Input: dimensioned drawing with shaded views. Units: mm. Origin: part minimum x, y, z. A direction names the side the tool comes from. Round coordinates to 2 decimals unless told otherwise and drop trailing zeros. Loops run counter-clockwise (first coordinate to the right, second up) from the corner with the lowest first, then second, coordinate; pieces in that order, holes last. Notation, with made-up numbers: (45.25, 18) - (54.25, 18) arc R28 cw to (54.25, 46) - close; hole circle Ø4 at (86.5, 70). An arc over 180 degrees is marked (long way). Answer as CSV lines item,"result".
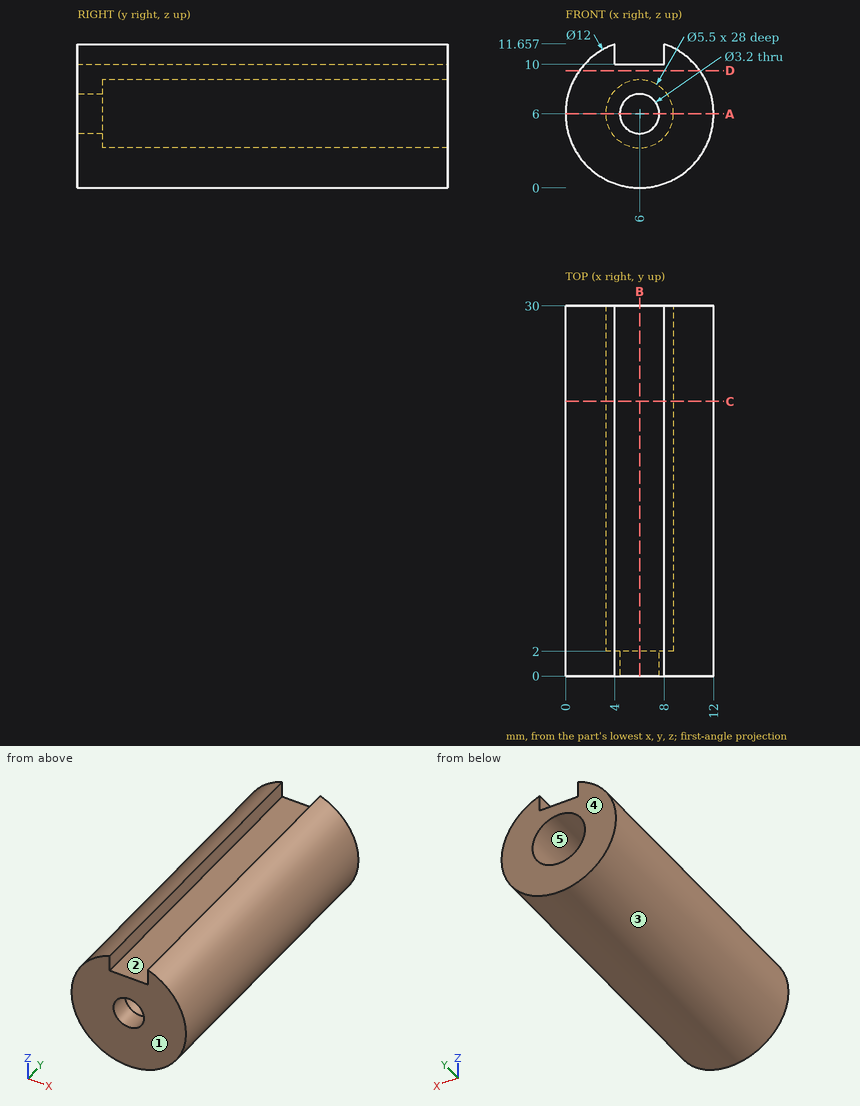
(1) Material intervals for line 1 along Z through (x, y) = (6, 1.1); line 2 along Z through (x, y) = (6, 11.5); line 3 along Y through (x, z) = (4, 7.75), sorted ascending.
Findings below:
line 1,"0 to 4.4, 7.6 to 10"
line 2,"0 to 3.25, 8.75 to 10"
line 3,"0 to 2"
(2) Pin query (flat end, axial travel): P1, Ø5, axis at x = 3, y = 4, coming from the +Z side; P2, Ø0.8, axis at y = 16.5, z = 11, coming from the -X side; P3, Ø5, axis at y = 12, z = 9, coming from the +X side; P4, Ø1.5, axis at x = 6.5, y = 12.5, coming from the -Z side. Return the tip coordinate at first contact, or that it passes through.
Findings below:
P1,"z = 11.66"
P2,"x = 2.15"
P3,"x = 11.98"
P4,"z = 0"
(3) Section D-D (z = 9.5). Output: boundary loops of the cut face in (x, y).
Findings below:
outline,"(1.13, 0) - (10.87, 0) - (10.87, 30) - (1.13, 30) - close"
(4) Draft query along Z for the marked faces 3, 4 and 5. Return one class per face: pulls with the +Z half, pulls with the -Z half, needs draft (parallel to the pull), parting line crosses it, or undercut.
Findings below:
face 3,"parting line crosses it"
face 4,"needs draft"
face 5,"undercut"
(5) Section C-C (y = 22.25). Output: boundary loops of the cut face in (x, z), and give its area (3 significant figures).
Findings below:
outline,"(4, 10) - (4, 11.66) arc R6 ccw (long way) to (8, 11.66) - (8, 10) - close; hole circle Ø5.5 at (6, 6)"
area,"81.8 mm2"
(6) Access query for the marked faces 1 and 2. Directions: +Z, -Z, +X, -X, +Y, -Y. A direction counts if a zero-diameter tool reaches every point of the face in a straight line with its end or side. Return the directions, or none.
Findings below:
face 1,"+Z, -Z, +X, -X, -Y"
face 2,"+Z, +Y, -Y"
(7) Section A-A (z = 6). Output: boundary loops of the cut face in (x, y), and give its area (3 significant figures).
Findings below:
outline,"(0, 0) - (4.4, 0) - (4.4, 2) - (3.25, 2) - (3.25, 30) - (0, 30) - close; (7.6, 0) - (12, 0) - (12, 30) - (8.75, 30) - (8.75, 2) - (7.6, 2) - close"
area,"200 mm2"
(8) Section B-B (x = 6). Output: boundary loops of the cut face in (y, z).
Findings below:
outline,"(0, 0) - (30, 0) - (30, 3.25) - (2, 3.25) - (2, 4.4) - (0, 4.4) - close; (0, 7.6) - (2, 7.6) - (2, 8.75) - (30, 8.75) - (30, 10) - (0, 10) - close"
